Input: part model. Units: mm. Frame: model coordinates. Face numbers are marked on the shaded views. Coordinates: 2 decimals unless noted, no trailing zeros. Write each loop counter-clockwise with the first axis right and the second up, starting at its lowest first coordinate (ties: lowest second). Pieces come first, ordered by that corner, then holes. Notation, with made-up numbers: (-9, -11.75) - (22, -11.75) arc R16 ccw to (22, 15.25) - close; hole circle Ø4 at (47.5, 76.25). An arc over 180 degrees is marked (long way). Use a Markdown table: item, result. Add a question column.
Q1. Material intervals for probe 1 along Y at (x, z) = (-60, 47); probe 2 along X at (y, z) = (-35.5, 11.5); probe 3 along X at (y, z) = (-26, 44), sorted ascending. Write a range as from..to.
Q2. Section query B-B (x = -78.5). Return the cut outline in (y, z).
Q3. Mould query, pull axis X, two halves, no side actions, for the marked faces 1, 2 and 3. Classes: released by +X, released by -X, zero draft, split by the parting line, or undercut.
Q4. Section query D-D (y = -86). Return the cut outline in (x, z), then the cut area to 3 significant figures.
Q5. Section query A-A (y = -28). Return the cut outline in (x, z), then the cut area to 3 significant figures.
Q6. Section query C-C (z = 41.5). Return the cut outline in (x, y).
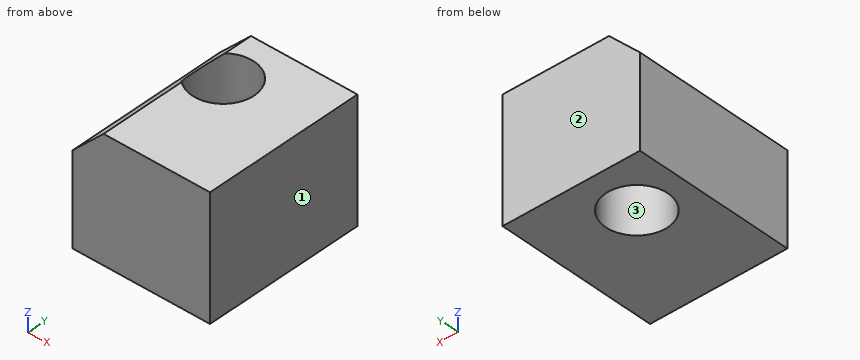
from build123d import *

# Parameters (mm, degrees)
F0_W        = 112.5368224457
F0_H        = 100.0910364091
F1_DEPTH    = 132.68445
F3_D        = 50.8
F4_T1_DEPTH = 263.3259457887


# Not quite as in the source:
# - a fillet or chamfer that OpenCascade refuses, or shapes differently, is made with other operations: its cross-section is extruded or revolved along the edge and cut away or added


with BuildPart() as f1:
    # F0 (on Front) → F1 (new body)
    with BuildSketch(Plane.XZ):
        with Locations((-44.0393215977, 6.0430746526)):
            Rectangle(F0_W, F0_H)
    extrude(amount=F1_DEPTH)

    # F3 (through all)
    with Locations(Plane(origin=(0, 0, -44.002443552), x_dir=(1, 0, 0), z_dir=(0, 0, -1))):
        with Locations((-58.6555227637, 42.9257005453)):
            Hole(F3_D / 2)

    # F4: chamfer of 25.4 on 1 edges, made by hand

    # F4_s2 → F4_t1 (cut)
    with BuildSketch(Plane.XZ.offset(-65.3207478943)):
        Polygon((-74.9077328205, 56.0885928571), (-100.3077328205, 30.6885928571), (-100.3077328205, 56.0885928571), align=None)
    extrude(amount=F4_T1_DEPTH, mode=Mode.SUBTRACT)


solid = f1.part
Values follow:
| question | item | result |
|---|---|---|
| 1 | probe 1 | -132.68..-68.29, -17.56..0 |
| 1 | probe 2 | -100.31..-82.95, -34.37..12.23 |
| 1 | probe 3 | -87..-77.59, -39.72..12.23 |
| 2 | outline | (-132.68, -44) - (-58.78, -44) - (-58.78, 52.5) - (-132.68, 52.5) - close; (-27.07, -44) - (0, -44) - (0, 52.5) - (-27.07, 52.5) - close |
| 3 | face 1 | released by +X |
| 3 | face 2 | zero draft |
| 3 | face 3 | undercut |
| 4 | outline | (-100.31, -44) - (12.23, -44) - (12.23, 56.09) - (-74.91, 56.09) - (-100.31, 30.69) - close |
| 4 | area | 10,900 mm2 |
| 5 | outline | (-100.31, -44) - (-79.21, -44) - (-79.21, 51.79) - (-100.31, 30.69) - close; (-38.1, -44) - (12.23, -44) - (12.23, 56.09) - (-38.1, 56.09) - close |
| 5 | area | 6,840 mm2 |
| 6 | outline | (-89.5, -132.68) - (12.23, -132.68) - (12.23, 0) - (-89.5, 0) - close; hole circle Ø50.8 at (-58.66, -42.93) |
